Input: part model. Units: mm. Frame: model coordinates. Coordinates: 2 decimals unless noted, no trailing zeros. Order: outer loops, then holes, each group sorted by start corner. A loop starts at its lowest first (then second) coordinate and runs counter-clockwise, first axis right, second up. Notation, with made-up numbers: (54, 71.5) -> (96, 71.5) arc R16 ccw to (96, 90.5) -> close; hole circle Ø5 at (59.25, 34). An arc over 180 degrees is marked (long way). Answer as CSV lines item,"result".
from build123d import *

# Parameters (mm, degrees)
SKETCH1_W           = 8.2
SKETCH1_H           = 8.2
SKETCH1_W_2         = 8
SKETCH1_H_2         = 8
BOSS_EXTRUDE1_DEPTH = 1.7
BOSS_EXTRUDE2_DEPTH = 1.5
CIRPATTERN1_COUNT   = 4
BOSS_EXTRUDE3_DEPTH = 0.1
SKETCH4_W           = 1.6
SKETCH4_H           = 1.2
BOSS_EXTRUDE4_DEPTH = 0.1


with BuildPart() as part:
    # Sketch1 → Boss-Extrude1 (new body)
    with BuildSketch(Plane(origin=(0, 0, 0), x_dir=(1, 0, 0), z_dir=(0, 1, 0))):
        Rectangle(SKETCH1_W, SKETCH1_H)
        Rectangle(SKETCH1_W_2, SKETCH1_H_2, mode=Mode.SUBTRACT)
    extrude(amount=BOSS_EXTRUDE1_DEPTH)

    # Sketch2 → Boss-Extrude2 (add, symmetric)
    with BuildSketch(Plane.ZY):
        with BuildLine():
            Line((6.115237938, -2.222344719), (4.246446609, -0.353553391))
            ThreePointArc((4.246446609, -0.353553391), (4.138060234, -0.191341716), (4.1, 0))
            Line((4.1, 0), (4.1, 0.022895615))
            Line((4.1, 0.022895615), (4, 0.022895615))
            Line((4, 0.022895615), (4, 0))
            ThreePointArc((4, 0), (4.04567228, -0.229610059), (4.175735931, -0.424264069))
            Line((4.175735931, -0.424264069), (6.04452726, -2.293055398))
            Line((6.04452726, -2.293055398), (6.115237938, -2.222344719))
        make_face()
    boss_extrude2 = extrude(amount=BOSS_EXTRUDE2_DEPTH, both=True)

    # CirPattern1: Boss-Extrude2 ×4 about axis
    cirpattern1_axis = Axis((0, 0, 0), (0, 1, 0))
    for i in range(1, CIRPATTERN1_COUNT):
        add(boss_extrude2.rotate(cirpattern1_axis, i * 360 / CIRPATTERN1_COUNT))

    # Sketch3 → Boss-Extrude3 (add)
    with BuildSketch(Plane(origin=(0, 1.7, 0), x_dir=(1, 0, 0), z_dir=(0, 1, 0))):
        Polygon((-4, -3.6), (-5.4, -3.6), (-7, -3.6), (-7, -0.1), (-7.400115841, -0.1), (-7.400115841, 2.4), (-7, 2.4), (-5.4, 2.4), (-5.000115841, 2.4), (-5.000115841, -0.1), (-5.4, -0.1), (-5.4, -2), (-4, -2), align=None)
    extrude(amount=BOSS_EXTRUDE3_DEPTH)

    # Sketch4 → Boss-Extrude4 (add)
    with BuildSketch(Plane(origin=(0, 1.7, 0), x_dir=(1, 0, 0), z_dir=(0, 1, 0))):
        with Locations((-1.8, -4.6)):
            Rectangle(SKETCH4_W, SKETCH4_H)
        with Locations((1.819415949, -4.6)):
            Rectangle(SKETCH4_W, SKETCH4_H)
    extrude(amount=BOSS_EXTRUDE4_DEPTH)


solid = part.part
1. Cut plane C-C (y = 1.2). Return the cut outline in (x, z).
Findings:
outline,"(-4.1, -4.1) -> (4.1, -4.1) -> (4.1, 4.1) -> (-4.1, 4.1) -> close; hole (-4, -4) -> (4, -4) -> (4, 4) -> (-4, 4) -> close"
2. Ray query, line 1 along X through (y, z) = (-1.7, -5.5). Return the intervals inside material, ascending.
Findings:
line 1,"x = -1.5 to 1.5"
3. Cut plane D-D (z = -3.75). Return the cut outline in (x, y), plus the area to 3 significant figures.
Findings:
outline,"(-4.1, 0) -> (-4, 0) -> (-4, 1.7) -> (-4.1, 1.7) -> close; (4, 0) -> (4.1, 0) -> (4.1, 1.7) -> (4, 1.7) -> close"
area,"0.340 mm2"
4. Cut plane A-A (x = 2.25). Return the cut outline in (y, z).
Findings:
outline,"(0, -4.1) -> (1.7, -4.1) -> (1.7, -4) -> (0, -4) -> close; (0, 4) -> (1.8, 4) -> (1.8, 5.2) -> (1.7, 5.2) -> (1.7, 4.1) -> (0, 4.1) -> close"
5. Cut plane B-B (z = -0.5). Return the cut outline in (x, y), plus the area to 3 significant figures.
Findings:
outline,"(-7.4, 1.7) -> (-5, 1.7) -> (-5, 1.8) -> (-7.4, 1.8) -> close; (-6.12, -2.22) -> (-6.04, -2.29) -> (-4.18, -0.42) arc R0.6 ccw to (-4, 0) -> (-4, 1.7) -> (-4.1, 1.7) -> (-4.1, 0) arc R0.5 cw to (-4.25, -0.35) -> close; (4, 0) arc R0.6 ccw to (4.18, -0.42) -> (6.04, -2.29) -> (6.12, -2.22) -> (4.25, -0.35) arc R0.5 cw to (4.1, 0) -> (4.1, 1.7) -> (4, 1.7) -> close"
area,"1.19 mm2"
6. Contact query for flat-ended pins moving along their axis: pin 1 (0.6 mm diameter, centred on x = 5.5, y = -1.5, fed in from +Z); pin 2 (0.5 mm diameter, centred on x = 1.5, y = 0.5, fed in from -Z); pin 3 (1.4 mm diameter, centred on x = 1.5, y = 0.5, fed in from +Z); pin 4 (4 mm diameter, centred on x = 4.5, z = 4, fed in from +Y). Output: stop coordinate, or through.
Findings:
pin 1,"stops at z = 1.5"
pin 2,"stops at z = -4.1"
pin 3,"stops at z = 4.14"
pin 4,"stops at y = 1.8"
